Input: part model. Units: mm. Frame: model coordinates. Give positions to 0.01 mm unless a question says otherwise; leave off trailing zeros. Loops run counter-clockwise (first coordinate to the right, second up) from the corner with the lowest first, then second, coordinate; pieces in that order, holes last. Notation, with made-up numbers: M 5.5,-33 L 48.5,-33 A24 ccw 48.5,2 Z; hole C -6,-0.5 d2. An arc over 180 degrees is marked long. Answer as a JSON object with one key per item and string values. Group by question number.
```python
from build123d import *

# Parameters (mm, degrees)
F0_W     = 3.175
F0_H     = 12.7
F4_DEPTH = 25.4


with BuildPart() as f1:
    # F0 (on Front) → F1 (revolve)
    with BuildSketch(Plane.XZ):
        Polygon((-3.175, 0), (0, 0), (0, 25.4), (-14.490464, 20.426942), (-7.480035, 0), align=None)
        with Locations((-1.5875, -6.35)):
            Rectangle(F0_W, F0_H)
    revolve(axis=Axis((0, 0, 12.7), (0, 0, 1)))

    # F3 (on offset) → F4 (cut)
    with BuildSketch(Plane.XY.offset(25.4)):
        Polygon((-2.321808, 17.121961), (0, 13.217989), (2.321808, 17.121961), align=None)
        Polygon((5.361183, 12.081927), (9.066876, 14.70864), (4.822371, 16.592079), align=None)
        Polygon((9.800797, 8.869025), (14.253382, 9.766958), (11.137602, 13.210079), align=None)
        Polygon((12.555691, 4.13157), (16.989782, 3.14637), (15.538319, 7.557313), align=None)
        Polygon((13.152306, -1.316087), (16.805701, -4.015067), (17.268056, 0.605473), align=None)
        Polygon((11.488088, -6.537513), (13.732781, -10.486329), (16.029476, -6.450445), align=None)
        Polygon((7.849109, -10.635165), (8.299245, -15.155028), (12.035488, -12.397556), align=None)
        Polygon((2.860897, -12.90467), (1.439099, -17.218634), (5.972642, -16.213571), align=None)
        Polygon((-2.619094, -12.95591), (-5.668423, -16.322418), (-1.116878, -17.242533), align=None)
        Polygon((-7.648871, -10.780075), (-11.801563, -12.620438), (-8.014412, -15.307565), align=None)
        Polygon((-11.363835, -6.751184), (-15.906058, -6.74905), (-13.534297, -10.741283), align=None)
        Polygon((-13.125397, -1.56179), (-17.276358, 0.282475), (-16.727686, -4.328613), align=None)
        Polygon((-12.630751, 3.896071), (-15.676916, 7.265443), (-17.045646, 2.82813), align=None)
        Polygon((-9.964925, 8.684211), (-11.382668, 12.999508), (-14.433521, 9.498728), align=None)
        Polygon((-5.586164, 11.979567), (-5.131781, 16.499005), (-9.340326, 14.536528), align=None)
    extrude(amount=-F4_DEPTH, mode=Mode.SUBTRACT)


solid = f1.part
```
1. Section B-B (z = 3). Output: boundary loops of the cut face in (x, y), then the cut area to 3 significant figures.
2. First-contact query: P1, Ø5, axis at x = 7.5, z = 6.5, coming from the -Y side; P2, Ø4, axis at x = 4.5, y = -3, coming from the +Z side; P3, Ø3, axis at x = -11.5, y = -1.5, coming from the +Z side; P4, Ø10, axis at x = 2, y = 3, coming from the +Z side. Flat tips, straight axial feed; report the tip coordinate or a pass-through.
3. Section A-A (z = -1). Output: boundary loops of the cut face in (x, y) (3 decimals).
4. Mould query, pull axis Y, two halves, no side actions, for faces 1 (the conical face through (0.2, 0.88, 25.09)), 2 (the flat face through (12.941, 4.046, 19.281)). Classes: pulls with the +Y half, pulls with the -Y half, needs draft (parallel to the pull), parting line crosses it, or undercut.
5. Material intervals for L1, parallel to Y at x = 3, z = 14.5; L2, parallel to Y at x = -0.25, z = -9; L3, parallel to Z at x = -6.25, y = 7, sorted ascending.
Geometry results:
{
 "1": {"outline": "C 0,0 d17.02", "area": "227 mm2"},
 "2": {"P1": "y = -8.63", "P2": "z = 24.23", "P3": "z = 21.93", "P4": "z = 25.4"},
 "3": {"outline": "C 0,0 d6.35"},
 "4": {"face 1": "parting line crosses it", "face 2": "undercut"},
 "5": {"L1": "-12.09 to 12.09", "L2": "-3.17 to 3.17", "L3": "5.55 to 22.18"}
}
